Can you work these out from the model? Positions are in its coordinate system, mm. A direction names the side the tool comes from. Coordinates: 2 decimals unless noted, no trailing zeros. Order: outer loops, then holes, each group sorted by start corner. A loop starts at its lowest first (then second) coordinate and runs counter-clockwise, first axis right, second up. Notation, with made-up numbers: (14, -2) - (22, -2) arc R20 ccw to (22, 25) - close; hole circle Ø1 at (31, -35.75). An arc over 180 degrees is marked (long way). Return JSON: item names as keys, results as strings. Group by question number.
1) If we mould it in two halves opening along X, with no side actions, what happens to faces 1 (the face through (22, -0.3, 2.5)), 2 (the face through (-9.2, 0, 6)), 3 (the face through (4, 6, 7)), 4 (the face through (-6, 4, 7))? For each: pulls with the +X half, pulls with the -X half, needs draft (parallel to the pull), parting line crosses it, or undercut.
2) Imagine slicing it at B-B (x = -6). Write out the boundary of the cut face in (y, z).
3) Which directions (+Z, -Z, +X, -X, +Y, -Y) give clear straight access to the entire face, cutting with the end or side of a thin tool? Please do faces 5 (the face through (0.31, 21.43, 0.6)), 6 (the face through (0, -9.2, 6)), 7 (the face through (-6, -4, 7)).
4) Imagine slicing it at C-C (y = -11.5). Write out the boundary of the cut face in (x, z).
5) Imagine slicing it at A-A (z = 4). Write out the boundary of the cut face in (x, y), and give its area (3 significant figures).
6) If I drill on line 1 along X through (y, z) = (6, 9.75); line 2 along Y through (x, z) = (-5.5, 7.5); line 3 along Z through (x, y) = (-15, -1.5), over which ranges is the centre line in solid material (lowest first)?
7) For pin 1 Ø5 at (y, z) = (-0.5, 7) entering from -X; pin 2 Ø5 at (x, z) = (-0.5, 7.5) entering from +Y; pin 3 Ø1 at (x, y) = (-3, 10) entering from +Z, each with a flat end and sliding along its axis, tell me the tip position at first contact or that it passes through.
```python
from build123d import *

# Parameters (mm, degrees)
SKETCH_W     = 44
SKETCH_H     = 44
PAD_DEPTH    = 3
SKETCH001_W  = 18.4
SKETCH001_H  = 18.4
PAD001_DEPTH = 7
POCKET_DEPTH = 7
FILLET_R     = 2
CHAMFER_SIZE = 0.5


with BuildPart() as part:
    # Sketch → Pad (new body)
    with BuildSketch(Plane.XY):
        Rectangle(SKETCH_W, SKETCH_H)
    extrude(amount=PAD_DEPTH)

    # Sketch001 (on Face6 of Pad) → Pad001 (join)
    with BuildSketch(Plane.XY.offset(3)):
        Rectangle(SKETCH001_W, SKETCH001_H)
    extrude(amount=PAD001_DEPTH)

    # Sketch002 (on Face11 of Pad001) → Pocket (cut)
    with BuildSketch(Plane.XY.offset(10)):
        Polygon((-9.2, 7.2), (-2, 0), (-9.2, -7.2), (-9.2, -9.2), (-7.2, -9.2), (0, -2), (7.2, -9.2), (9.2, -9.2), (9.2, -7.2), (2, 0), (9.2, 7.2), (9.2, 9.2), (7.2, 9.2), (0, 2), (-7.2, 9.2), (-9.2, 9.2), align=None)
    extrude(amount=-POCKET_DEPTH, mode=Mode.SUBTRACT)

    # Fillet
    fillet_edges = [part.edges().sort_by_distance(p)[0] for p in [
        (0, -22, 0),
        (-22, 0, 0),
        (0, 22, 0),
        (22, 0, 0),
    ]]
    fillet(fillet_edges, radius=FILLET_R)

    # Chamfer
    chamfer_edges = [part.edges().sort_by_distance(p)[0] for p in [
        (0, 9.2, 10),
        (-9.2, 0, 10),
        (0, -9.2, 10),
        (9.2, 0, 10),
    ]]
    chamfer(chamfer_edges, length=CHAMFER_SIZE)


solid = part.part
```
Calculated:
{
 "1": {"face 1": "pulls with the +X half", "face 2": "pulls with the -X half", "face 3": "undercut", "face 4": "undercut"},
 "2": {"outline": "(-22, 2) arc R2 ccw to (-20, 0) - (20, 0) arc R2 ccw to (22, 2) - (22, 3) - (9.2, 3) - (9.2, 9.5) - (8.7, 10) - (8, 10) - (8, 3) - (4, 3) - (4, 10) - (-4, 10) - (-4, 3) - (-8, 3) - (-8, 10) - (-8.7, 10) - (-9.2, 9.5) - (-9.2, 3) - (-22, 3) - close"},
 "3": {"face 5": "-Z, +X, -X, +Y", "face 6": "+Z, +X, -X, -Y", "face 7": "+Z"},
 "4": {"outline": "(-22, 2) arc R2 ccw to (-20, 0) - (20, 0) arc R2 ccw to (22, 2) - (22, 3) - (-22, 3) - close"},
 "5": {"outline": "(-9.2, -7.2) - (-2, 0) - (-9.2, 7.2) - close; (-7.2, -9.2) - (7.2, -9.2) - (0, -2) - close; (-7.2, 9.2) - (0, 2) - (7.2, 9.2) - close; (2, 0) - (9.2, -7.2) - (9.2, 7.2) - close", "area": "207 mm2"},
 "6": {"line 1": "-8.95 to -8, -4 to 4, 8 to 8.95", "line 2": "-9.2 to -7.5, -3.5 to 3.5, 7.5 to 9.2", "line 3": "0 to 3"},
 "7": {"pin 1": "x = -9.2", "pin 2": "y = 9.2", "pin 3": "z = 3"}
}
